Part model, mm, in its own coordinate system. Face numbers are marked on the shaded views. A direction names the side the tool comes from. Coordinates: 2 decimals unless noted, no trailing zeros. Write each loop counter-clockwise with the first axis right and the second up, starting at its lowest first coordinate (ties: lowest second). Pieces come first, ordered by that corner, then holes. Notation, with made-up numbers: (44.25, 4.5) -> (80.25, 4.5) arc R29 cw to (80.25, 32.5) -> close; hole circle Ø6 at (76.5, 25.25). An arc over 180 degrees is marked (long way). Write item = value, one per line.
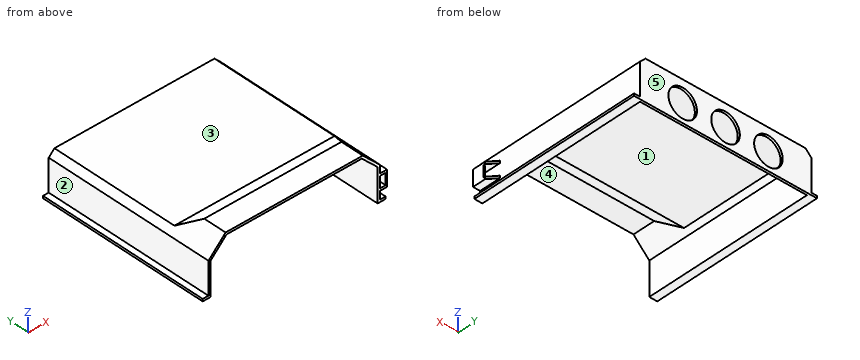
from build123d import *

# Parameters (mm, degrees)
F0_W        = 150
F0_H        = 45
F1_DEPTH    = 150
F2_W        = 5
F2_H        = 150
F3_DEPTH    = 2
F5_DEPTH    = 150
F6_SIZE     = 15
F7_T        = 2
F7_T3_DEPTH = 154
F7_T5_DEPTH = 144
F8_R        = 12.5
F9_DEPTH    = 25
F11_DEPTH   = 10
F13_DEPTH   = 14
F14_W       = 5
F14_H       = 10
F15_DEPTH   = 25
F16_W       = 1.2
F16_H       = 10
F16_W_2     = 1.4301043111
F17_DEPTH   = 6.2


# Not quite as in the source:
# - a shell that OpenCascade refuses in one call is made with other operations: the cavity is built on its own and cut out


with BuildPart() as f1:
    # F0 (on Front) → F1 (new body)
    with BuildSketch(Plane.XZ):
        with Locations((75, 22.5)):
            Rectangle(F0_W, F0_H)
    extrude(amount=F1_DEPTH)

    # F2 (on face) → F3 (join)
    with BuildSketch(Plane(origin=(0, 0, 0), x_dir=(1, 0, 0), z_dir=(0, 0, -1))):
        with Locations((152.5, 75)):
            Rectangle(F2_W, F2_H)
        with Locations((-2.5, 75)):
            Rectangle(F2_W, F2_H)
    extrude(amount=-F3_DEPTH)

    # F4 (on face) → F5 (cut, through all)
    with BuildSketch(Plane.YZ.offset(150)):
        Polygon((0, 35), (0, 45), (-130, 45), (-112.6794919243, 35), align=None)
    extrude(amount=-F5_DEPTH, mode=Mode.SUBTRACT)

    # F6
    f6_edges = [f1.edges().sort_by_distance(p)[0] for p in [
        (0, -140, 45),
        (150, -140, 45),
    ]]
    chamfer(f6_edges, length=F6_SIZE)

    # F7: shell of thickness 2, made by hand


with BuildPart() as f7_core1:
    # F7_t2: copy of F1
    add(f1.part)

    # the walls: a layer under each face that stays
    f7_faces = [f7_core1.faces().sort_by_distance(p)[0] for p in [
        (0, -75, 16),
        (75, 0, 17.5),
        (2.5, -25, 32.5),
        (-2.5, -75, 2),
        (75, -56.3397459622, 35),
        (147.5, -25, 32.5),
        (150, -75, 16),
        (152.5, -75, 2),
        (155, -75, 1),
        (-5, -75, 1),
        (75, -121.3397459622, 40),
        (75, -140, 45),
    ]]
    thicken(f7_faces, amount=-F7_T, mode=Mode.SUBTRACT)

    # F7_s4 → F7_t3 (cut)
    with BuildSketch(Plane.XZ.offset(-2)):
        Polygon((-0.02, 2.02), (2, 2), (2, 0), (0, 0), align=None)
        Polygon((150.02, 2.02), (148, 2), (148, 0), (150, 0), align=None)
    extrude(amount=F7_T3_DEPTH, mode=Mode.SUBTRACT)

    # F7_s6 → F7_t5 (cut)
    with BuildSketch(Plane.YZ.offset(3)):
        Polygon((-112.6694919243, 35.0373205081), (-112.6794919243, 33), (-113.2153903092, 33), (-113.6794919243, 33.2679491924), align=None)
    extrude(amount=F7_T5_DEPTH, mode=Mode.SUBTRACT)


with BuildPart() as f1_1:
    add(f1.part)

    # what is left inside the walls is the cavity
    f7_cavity = [f7_core1.part.solids().sort_by_distance(p)[0] for p in [
        (75, -100.666667, 0.02),
    ]]
    add(f7_cavity, mode=Mode.SUBTRACT)

    # F8 (on face) → F9 (cut)
    with BuildSketch(Plane(origin=(0, 0, 0), x_dir=(-1, 0, 0), z_dir=(0, 1, 0))):
        with Locations((-112.5, 16)):
            Circle(F8_R)
        with Locations((-75, 16)):
            Circle(F8_R)
        with Locations((-37.5, 16)):
            Circle(F8_R)
    extrude(amount=-F9_DEPTH, mode=Mode.SUBTRACT)

    # F10 (on face) → F11 (join)
    with BuildSketch(Plane.XZ.offset(150)):
        Polygon((156.2, 9), (156.2, 23), (150, 23), (150, 21), (155, 21), (155, 11), (150, 11), (150, 9), align=None)
    extrude(amount=-F11_DEPTH)

    # F12 (on face) → F13 (join, through all)
    with BuildSketch(Plane.XY.offset(23)):
        Polygon((150, -140), (156.2, -140), (156.2, -138.8), (150, -131.4111277259), align=None)
    extrude(amount=-F13_DEPTH)

    # F14 (on face) → F15 (cut)
    with BuildSketch(Plane.XZ.offset(150)):
        with Locations((152.5, 16)):
            Rectangle(F14_W, F14_H)
    extrude(amount=-F15_DEPTH, mode=Mode.SUBTRACT)

    # F16 (on face) → F17 (cut, through all)
    with BuildSketch(Plane.YZ.offset(156.2)):
        with Locations((-139.4, 16)):
            Rectangle(F16_W, F16_H)
        with Locations((-138.0849478444, 16)):
            Rectangle(F16_W_2, F16_H)
    extrude(amount=-F17_DEPTH, mode=Mode.SUBTRACT)


solid = f1_1.part
Q1. Saw through at B-B on y = -91. Give the cut face in (x, z), and give its area (3 significant figures).
Model answer:
outline = (-5, 0) -> (2, 0) -> (2, 29.17) -> (5.83, 33) -> (144.17, 33) -> (148, 29.17) -> (148, 0) -> (155, 0) -> (155, 2) -> (150, 2) -> (150, 30) -> (145, 35) -> (5, 35) -> (0, 30) -> (0, 2) -> (-5, 2) -> close
area = 442 mm²
Q2. Saw through at D-D on z = 26.5. Give the cut face in (x, y), and give its area (3 significant figures).
Model answer:
outline = (0, -150) -> (2, -150) -> (2, -2) -> (30.72, -2) -> (30.72, 0) -> (0, 0) -> close; (44.28, -2) -> (68.22, -2) -> (68.22, 0) -> (44.28, 0) -> close; (81.78, -2) -> (105.72, -2) -> (105.72, 0) -> (81.78, 0) -> close; (119.28, -2) -> (148, -2) -> (148, -150) -> (150, -150) -> (150, 0) -> (119.28, 0) -> close
area = 811 mm²
Q3. Saw through at C-C on x = 112.5. Give the cut face in (y, z), and give its area (3 significant figures).
Model answer:
outline = (-150, 43) -> (-130.54, 43) -> (-113.22, 33) -> (-2, 33) -> (-2, 28.5) -> (0, 28.5) -> (0, 35) -> (-112.68, 35) -> (-130, 45) -> (-150, 45) -> close; (-2, 0) -> (0, 0) -> (0, 3.5) -> (-2, 3.5) -> close
area = 321 mm²
Q4. Pin check, flat tips, straight feed: pin 1 (15 mm diameter, centred on x = 37.5, z = 16, fed in from +Y); pin 2 (1 mm diameter, centred on x = 116.5, y = -44.5, fed in from -Z); pin 3 (4 mm diameter, centred on x = 152.5, y = -38, fed in from +Z); pin 4 (23.5 mm diameter, centred on y = -109.5, z = 13, fed in from +X). Stop position of each tip, or through.
Model answer:
pin_1 = through
pin_2 = 33
pin_3 = 2
pin_4 = 155
Q5. Saw through at A-A on z = 16. Give the cut face in (x, y).
Model answer:
outline = (0, -150) -> (2, -150) -> (2, -2) -> (25, -2) -> (25, 0) -> (0, 0) -> close; (50, -2) -> (62.5, -2) -> (62.5, 0) -> (50, 0) -> close; (87.5, -2) -> (100, -2) -> (100, 0) -> (87.5, 0) -> close; (125, -2) -> (148, -2) -> (148, -150) -> (150, -150) -> (150, 0) -> (125, 0) -> close; (155, -150) -> (156.2, -150) -> (156.2, -140) -> (155, -140) -> close
Q6. Which spindle directions (+Z, -Z, +X, -X, +Y, -Y) get a long thin tool onto all of the face, cutting with end or side? Do the marked faces 4 and 5. Say none if no direction does.
Model answer:
face_4 = -Z, -Y
face_5 = +Z, -Z, +X, -X, +Y
Q7. Probe line 1 (Z direction, x = 37.5, y = -1.15); line 2 (X direction, y = -125, z = 21); line 3 (Z direction, x = 77, y = -102.5). List the from-to ranges inside material, lowest first. Write a range as from..to.
Model answer:
line_1 = 0..3.5, 28.5..35
line_2 = 0..2, 148..150
line_3 = 33..35
Q8. Mould opens along X. For the marked faces 1, 2 and 3 say: released by +X, released by -X, zero draft, split by the parting line, or undercut.
Model answer:
face_1 = undercut
face_2 = released by -X
face_3 = zero draft
